Here's how the part is built. I have some questions about the finished solid (model axes, mm). Face numbers are marked on the shaded views. A direction names the side the tool comes from. Round coordinates to 2 decimals unless told otherwise and drop trailing zeros. Order: outer loops, then holes, each group sorted by start corner. A loop starts at its lowest first (then second) coordinate and runs counter-clockwise, first axis right, second up. Notation, with made-up numbers: (23, 26) -> (56, 26) arc R21 ccw to (56, 47) -> close; hole circle Ø2 at (-3, 25.25). An arc over 180 degrees is marked (long way). Use a Markdown table: item, result. Add a question column.
(1) Thinking about a two-plate mould opening in Y: for the marked faces 1, 2, 3 and 4, which applies, pulls with the +Y half, pulls with the -Y half, needs draft (parallel to the pull), parting line crosses it, or undercut?
(2) I want a section at B-B, the plane x = -20.5. Please give me the cut outline in (y, z), then the cut area to 3 significant figures.
(3) I'm going to push flat-ended pins straight in: P1, Ø1.8, axis at x = -21, z = 26, coming from the -Y side; P2, Ø6, axis at x = 9.5, z = 22.5, coming from the +Y side; P3, Ø3, axis at x = 22, z = 24.5, coming from the -Y side; P4, Ø12.5, axis at x = -18, y = 16.5, coming from the +Z side. Where does each tip first touch, or does it pass through?
(4) I want a section at D-D, the plane z = 12. Please give me the cut outline in (x, y), then the cut area to 3 significant figures.
(5) On a 3-axis mill with a long thin cutter (end or side, diameter ignored), from which of +Z, -Z, +X, -X, +Y, -Y can I reach the whole of each face in a straight line? I mean the marked faces 5, 6 and 7. Say none if no direction works.
(6) If I drill on probe 1 along X at (y, z) = (26.25, 26); probe 2 along Y at (x, z) = (5, 13); probe 3 along X at (y, z) = (2.25, -25), over which ranges is the centre line in solid material (lowest first)?
(7) I want a section at A-A, the plane y = 14. Please give me the cut outline in (x, z), then the cut area to 3 significant figures.
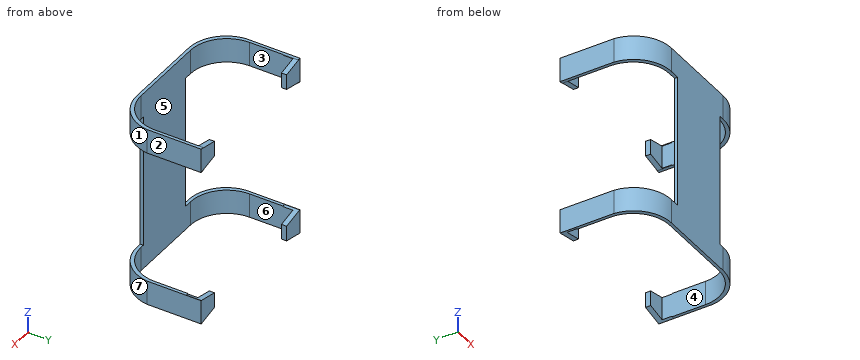
Autodesk Inventor part; units mm, degrees
ref_plane "YZ Plane" through (0, 0, 0) normal (1, 0, 0) x (0, 1, 0)
ref_plane "XZ Plane" through (0, 0, 0) normal (0, 1, 0) x (-1, 0, 0)
ref_plane "XY Plane" through (0, 0, 0) normal (0, 0, 1) x (1, 0, 0)
sketch "Sketch1" plane through (0, 0, 0) normal (0, 1, 0) x (-1, 0, 0)
  line L0 (-26, -31) -> (26, -31)
  line L1 (26, -31) -> (26, 31)
  line L2 (26, 31) -> (-26, 31)
  line L3 (-26, 31) -> (-26, -31)
  line L4 (-26, -31) -> (26, 31) construction
  line L5 (26, -31) -> (-26, 31) construction
  point P0 (0, 0)
  dimension "d0" = 52
  dimension "d2" = 62
extrude "Extrusion1" add sketch "Sketch1" along normal blind 1.02
sketch "Sketch2" plane through (0, 1.02, 0) normal (0, 1, 0) x (1, 0, 0)
  line L0 (26, 31) -> (-26, 31)
  line L1 (-26, 31) -> (-26, -31)
  line L2 (-26, -31) -> (26, -31)
  line L3 (-26, 31) -> (-25, 31)
  line L4 (-25, 31) -> (-25, -31)
  line L5 (-26, -31) -> (-25, -31)
  line L6 (-26, -31) -> (-26, 31)
  line L7 (0, 46.5401) -> (0, -49.8176) construction
  line L8 (26, 31) -> (26, -31)
  line L9 (26, 31) -> (25, 31)
  line L10 (25, 31) -> (25, -31)
  line L11 (26, -31) -> (25, -31)
  line L12 (26, -31) -> (26, 31)
  point P0 (0, 0)
  dimension "d5" = 1
extrude "Extrusion2" add sketch "Sketch2" along normal blind 28 contours L8 L2 L10 L0 | L4 L2 L1 L0
fillet "Fillet1" radius 12 1 edges at (-25, 1.02, 0)
mirror "Mirror1" about plane through (0, 0, 0) normal (1, 0, 0) of "Fillet1"
sketch "Sketch3" plane through (-26, 0, -31) normal (-1, 0, 0) x (0, 0, 1)
  line L0 (0, 0) -> (62, 0)
  line L1 (62, 29.02) -> (61, 29.02) construction
  line L2 (61, 29.02) -> (61, 27.32)
  line L3 (61, 27.32) -> (53, 27.32)
  line L4 (53, 27.32) -> (53, 29.02)
  line L5 (61, 29.02) -> (53, 29.02)
  line L6 (53, 29.02) -> (61, 29.02)
  point P0 (31, 0)
  dimension "d9" = 1
  dimension "d10" = 1.7
  dimension "d11" = 8
extrude "Extrusion3" add sketch "Sketch3" against normal blind 7
mirror "Mirror3" about plane through (0, 0, 0) normal (0, 0, 1) of "Extrusion3"
mirror "Mirror4" about plane through (0, 0, 0) normal (1, 0, 0) of "Extrusion3", "Mirror3"
sketch "Sketch6" plane through (0, 29.02, 0) normal (0, 1, 0) x (1, 0, 0)
  line L0 (-30.2809, -30.0039) -> (31.8564, -30.0039)
  line L1 (31.8564, -30.0039) -> (31.8564, -41.1164)
  line L2 (31.8564, -41.1164) -> (-30.2809, -41.1164)
  line L3 (-30.2809, -41.1164) -> (-30.2809, -30.0039)
  line L4 (-30.2809, 39.7218) -> (31.1002, 39.7218)
  line L5 (31.1002, 39.7218) -> (31.1002, 29.9909)
  line L6 (31.1002, 29.9909) -> (-30.2809, 29.9909)
  line L7 (-30.2809, 29.9909) -> (-30.2809, 39.7218)
  line L8 (-30.2809, 22.0008) -> (-10.2809, 22.0008)
  line L9 (-10.2809, 22.0008) -> (-10.2809, -21.9612)
  line L10 (-10.2809, -21.9612) -> (-30.2809, -21.9612)
  line L11 (-30.2809, -21.9612) -> (-30.2809, 22.0008)
  line L12 (31.8564, -21.9503) -> (11.8564, -21.9503)
  line L13 (11.8564, -21.9503) -> (11.8564, 22.0008)
  line L14 (11.8564, 22.0008) -> (31.8564, 22.0008)
  line L15 (31.8564, 22.0008) -> (31.8564, -21.9503)
  point P0 (0, 0)
  dimension "d26" = 20
  dimension "d27" = 20
extrude "Extrusion6" cut sketch "Sketch6" against normal through all
sketch "Sketch7" plane through (0, 29.02, 0) normal (0, 1, 0) x (1, 0, 0)
  line L0 (19, 22.0008) -> (19, 30)
  line L1 (26, 22.0008) -> (26, 29.9909)
  line L2 (19, 30) -> (19, 28.5)
  line L3 (19, 28.5) -> (26, 30)
  line L4 (19, 30) -> (26, 30)
  line L5 (19, 30) -> (19, 22.0008) construction
  line L6 (18.3, 25.9838) -> (30.5903, 25.9838) construction
  line L7 (19, 29.9668) -> (19, 21.9676)
  line L8 (26, 29.9668) -> (26, 21.9767)
  line L9 (19, 21.9676) -> (19, 23.4676)
  line L10 (19, 23.4676) -> (26, 21.9676)
  line L11 (19, 21.9676) -> (26, 21.9676)
  line L12 (19, 21.9676) -> (19, 29.9668) construction
  point P0 (0, 0)
  dimension "d30" = 1.5
extrude "Extrusion7" cut sketch "Sketch7" against normal blind 5
mirror "Mirror6" about plane through (0, 0, 0) normal (1, 0, 0) of "Extrusion7"
mirror "Mirror7" about plane through (0, 0, 0) normal (0, 0, 1) of "Extrusion7", "Mirror6"
sketch "Sketch8" plane through (-26, 0, 30.0039) normal (0, 0, 1) x (1, 0, 0)
  line L0 (0, 0) -> (0, 29.02)
  line L1 (52, 0) -> (0, 0)
  line L2 (51, 29.02) -> (52, 29.02)
  arc A0 (0, 13.6957) -> (12.3777, 0) centre (12.3777, 12.4411) ccw
  line L3 (0, 11.1866) -> (0, 0)
  arc A1 (1, 13.02) -> (13, 1.02) centre (13, 13.02) ccw
  line L4 (52, 29.02) -> (52, 0)
  line L5 (26, 0) -> (26, 62.522) construction
  line L6 (52, 0) -> (52, 29.02)
  line L7 (0, 0) -> (52, 0)
  arc A2 (39.6223, 0) -> (52, 13.6957) centre (39.6223, 12.4411) ccw
  line L8 (52, 11.1866) -> (52, 0)
  arc A3 (39, 1.02) -> (51, 13.02) centre (39, 13.02) ccw
  dimension "d35" = 0.5788
extrude "Extrusion8" cut sketch "Sketch8" against normal through all contours A2 L4 L1 | L0 A0 L1
properties part number "tapa"
Taken from the geometry:
| question | item | result |
|---|---|---|
| 1 | face 1 | pulls with the -Y half |
| 1 | face 2 | needs draft |
| 1 | face 3 | undercut |
| 1 | face 4 | undercut |
| 2 | outline | (2.07, -29.99) -> (3.65, -29.99) -> (3.65, -22) -> (2.07, -22) -> close; (2.07, 21.96) -> (3.65, 21.96) -> (3.65, 30) -> (2.07, 30) -> close; (27.32, -28.82) -> (29.02, -28.82) -> (29.02, -23.15) -> (27.32, -23.15) -> close; (27.32, 23.15) -> (29.02, 23.15) -> (29.02, 28.82) -> (27.32, 28.82) -> close |
| 2 | area | 44.6 mm2 |
| 3 | P1 | stops at y = 1.82 |
| 3 | P2 | stops at y = 1.02 |
| 3 | P3 | stops at y = 2.07 |
| 3 | P4 | passes through |
| 4 | outline | (-10.28, 0) -> (11.86, 0) -> (11.86, 1.02) -> (-10.28, 1.02) -> close |
| 4 | area | 22.6 mm2 |
| 5 | face 5 | +Z, -Z, +Y |
| 5 | face 6 | +Z, -Z |
| 5 | face 7 | +Z, -Z, +X, -Y |
| 6 | probe 1 | x = -26 to -25, 25 to 26 |
| 6 | probe 2 | y = 0 to 1.02 |
| 6 | probe 3 | x = -20.76 to -18.29, 18.29 to 20.76 |
| 7 | outline | (-26, -29.99) -> (-25, -29.99) -> (-25, -22) -> (-26, -22) -> close; (-26, 21.96) -> (-25, 21.96) -> (-25, 30) -> (-26, 30) -> close; (25, -29.99) -> (26, -29.99) -> (26, -22) -> (25, -22) -> close; (25, 21.95) -> (26, 21.95) -> (26, 30) -> (25, 30) -> close |
| 7 | area | 32.1 mm2 |
